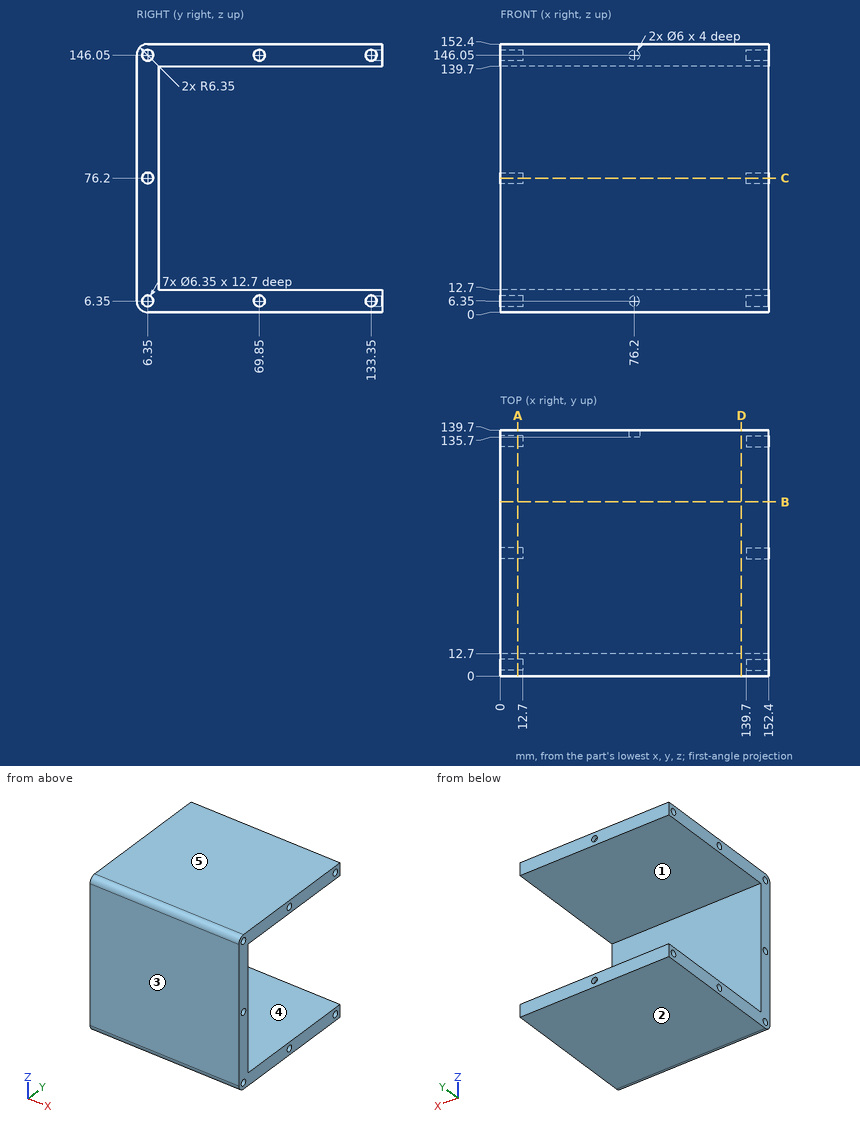
Verification items for this drawing (mm, ordinates from the low corner). A direction names the side the tool comes from. Coordinates: 2 decimals unless noted, no trailing zeros. Order: outer loops, then holes, each group sorted by start corner. A loop starts at its lowest first (then second) coordinate and runs counter-clockwise, first axis right, second up. Notation, with made-up numbers: (-29, 21) - (5, 21) arc R16 ccw to (5, 49) - close; hole circle Ø5 at (-7, 61.25). An arc over 180 degrees is marked (long way). Answer in a Markdown table with one row per item. Add a question column.
1. Section check A-A (x = 10). Enter the section's corners in (y, z) (3 decimals).
2. Section check B-B (y = 99). Enter the section's corners in (x, z), plus the area to 3 significant figures.
3. Access from +Z, -Z, +X, -X, +Y, -Y to the whole of each face (thin tool, end or side, straight path). Record for the marked faces 4 and 5.
4. Draft check along Z on the marked faces 1, 2 and 3. Enter one of: +Z half, -Z half, draft (parallel to the pull), parting line (faces both ways), or undercut.
5. Section check D-D (x = 137). Enter the section's corners in (y, z).
6. Material ranges on L1, parallel to Z at x = 142.5, y = 133.35 (3 decimals); L2, parallel to Y at x = 3.25, z = 146.05 (3 decimals); L3, parallel to Z at x = 117.5, y = 95, recorded low to high. Write a range as [from, to].
7. Gauge pin test, flat ends, axial feed: pin 1 Ø4 at (y, z) = (6.35, 76.2) entering from +X; pin 2 Ø10 at (x, z) = (135.5, 87.5) entering from +Y; pin 3 Ø3 at (y, z) = (134.5, 6.5) entering from -X. Record the tip position at first contact, or that the pin passes through.
8. Section check C-C (z = 76.2). Enter the section's corners in (x, y) (3 decimals).
Data:
| question | item | result |
|---|---|---|
| 1 | outline | (0, 6.35) arc R6.35 ccw to (6.35, 0) - (139.7, 0) - (139.7, 12.7) - (12.7, 12.7) - (12.7, 139.7) - (139.7, 139.7) - (139.7, 152.4) - (6.35, 152.4) arc R6.35 ccw to (0, 146.05) - close; hole circle Ø6.35 at (6.35, 6.35); hole circle Ø6.35 at (6.35, 76.2); hole circle Ø6.35 at (6.35, 146.05); hole circle Ø6.35 at (69.85, 6.35); hole circle Ø6.35 at (69.85, 146.05); hole circle Ø6.35 at (133.35, 6.35); hole circle Ø6.35 at (133.35, 146.05) |
| 2 | outline | (0, 0) - (152.4, 0) - (152.4, 12.7) - (0, 12.7) - close; (0, 139.7) - (152.4, 139.7) - (152.4, 152.4) - (0, 152.4) - close |
| 2 | area | 3,870 mm² |
| 3 | face 4 | +X, -X, +Y |
| 3 | face 5 | +Z, +X, -X, +Y, -Y |
| 4 | face 1 | undercut |
| 4 | face 2 | -Z half |
| 4 | face 3 | draft |
| 5 | outline | (0, 6.35) arc R6.35 ccw to (6.35, 0) - (139.7, 0) - (139.7, 12.7) - (12.7, 12.7) - (12.7, 139.7) - (139.7, 139.7) - (139.7, 152.4) - (6.35, 152.4) arc R6.35 ccw to (0, 146.05) - close |
| 6 | L1 | z = [0, 3.175], [9.525, 12.7], [139.7, 142.875], [149.225, 152.4] |
| 6 | L2 | y = [0, 3.175], [9.525, 66.675], [73.025, 130.175], [136.525, 139.7] |
| 6 | L3 | z = [0, 12.7], [139.7, 152.4] |
| 7 | pin 1 | stops at x = 139.7 |
| 7 | pin 2 | stops at y = 12.7 |
| 7 | pin 3 | stops at x = 12.7 |
| 8 | outline | (0, 0) - (152.4, 0) - (152.4, 3.175) - (139.7, 3.175) - (139.7, 9.525) - (152.4, 9.525) - (152.4, 12.7) - (0, 12.7) - (0, 9.525) - (12.7, 9.525) - (12.7, 3.175) - (0, 3.175) - close |
